Could you check a few things on this model? Use its own coordinates, in mm. Face numbers are marked on the shaded views. A direction names the side the tool comes from. Give positions to 0.01 mm unless a question says otherwise; leave off trailing zeros. Write each loop counter-clockwise with the first axis right and the second up, starting at its lowest first coordinate (ties: lowest second). Pieces come first, ordered by that corner, then holes. Notation, with made-up numbers: (49, 89) - (75, 89) arc R25 cw to (75, 116) - close; hole circle Ø8 at (-39.5, 13.25). An arc over 180 degrees is marked (long way). Use one line per item in the form item = value.
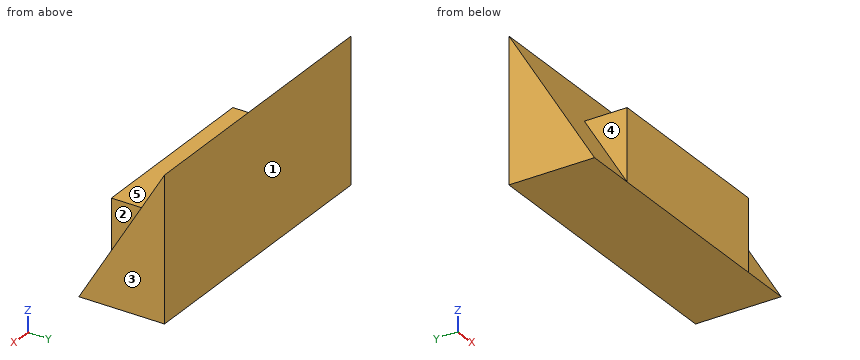
```python
from build123d import *

# Parameters (mm, degrees)
F1_DEPTH = 127
F2_START = 22.225
F2_DEPTH = 82.677


with BuildPart() as f1:
    # F0 (on Right) → F1 (new body)
    with BuildSketch(Plane.YZ):
        Polygon((30.5216386862, -38.4214240238), (30.5216386862, 25.0785759762), (11.4716386862, -6.6714240238), (-7.5783613138, -38.4214240238), align=None)
    extrude(amount=F1_DEPTH)

    # F0 (on Right) → F2 (join)
    with BuildSketch(Plane.YZ.offset(F2_START)):
        Polygon((-7.5783613138, -38.4214240238), (11.4716386862, -6.6714240238), (-7.5783613138, -6.6714240238), align=None)
    extrude(amount=F2_DEPTH)


solid = f1.part
```
1. For pin 1 (9.5 mm diameter, centred on y = 4, z = -25.5, fed in from -X); pin 2 (1 mm diameter, centred on x = 32, z = 13, fed in from -Y); pin 3 (8 mm diameter, centred on x = 28.5, z = 0.5, fed in from -Y); pin 4 (9.5 mm diameter, centred on x = 84, y = 3.5, fed in from +Z), each with a flat end and sliding along its axis, tell me the tip position at first contact or that it passes through.
Response values:
pin_1 = 0
pin_2 = 22.97
pin_3 = 13.37
pin_4 = -6.67
2. Imagine slicing it at B-B, the plane y = 10. List the corners of the cut face in (x, z) for me (3 decimals).
Response values:
outline = (0, -38.421) - (127, -38.421) - (127, -9.124) - (104.902, -9.124) - (104.902, -6.671) - (22.225, -6.671) - (22.225, -9.124) - (0, -9.124) - close
3. Which directions (+Z, -Z, +X, -X, +Y, -Y) give clear straight access to the entire face, cutting with the end or side of a thin tool? Please do the marked faces 1, 2, 3, 4 and 5.
Response values:
face_1 = +Z, -Z, +X, -X, +Y
face_2 = +Z, +X, -Y
face_3 = +Z, -Z, +X, +Y, -Y
face_4 = +Z, -X, -Y
face_5 = +Z, +X, -X, -Y
4. Imagine slicing it at A-A, the plane x = 34. List the corners of the cut face in (y, z) for me, and give its area (3 significant figures).
Response values:
outline = (-7.58, -38.42) - (30.52, -38.42) - (30.52, 25.08) - (11.47, -6.67) - (-7.58, -6.67) - close
area = 1,510 mm²
5. Imagine slicing it at C-C, the plane z = -22. List the corners of the cut face in (x, y) for me (1 decimal), and give its area (3 significant figures).
Response values:
outline = (0, 2.3) - (22.2, 2.3) - (22.2, -7.6) - (104.9, -7.6) - (104.9, 2.3) - (127, 2.3) - (127, 30.5) - (0, 30.5) - close
area = 4,400 mm²
6. If I drill on line 1 (Z direction, x = 56, y = 7.5); line 2 (Y direction, x = 25.5, z = 18); line 3 (Y direction, x = 75, z = 13.5), over which ranges is the centre line in solid material (lowest first)? Write a range as from..to.
Response values:
line_1 = -38.42..-6.67
line_2 = 26.27..30.52
line_3 = 23.57..30.52
7. Imagine slicing it at D-D, the plane x = 118.5. List the corners of the cut face in (y, z) for me.
Response values:
outline = (-7.58, -38.42) - (30.52, -38.42) - (30.52, 25.08) - close
